```python
from build123d import *

# Parameters (mm, degrees)
SKETCH002_R     = 2.5
PAD002_DEPTH    = 7.5
SKETCH003_R     = 2.5
PAD003_DEPTH    = 7.25
SKETCH004_W     = 7.7928
SKETCH004_H     = 28.3985
PAD004_DEPTH    = 7
SKETCH006_W     = 20.21794
SKETCH006_H     = 4
POCKET_DEPTH    = 3
SKETCH_R        = 1.6
PAD_DEPTH       = 2
SKETCH001_W     = 53.9946
SKETCH001_H     = 28.4007
SKETCH001_W_2   = 44.2
SKETCH001_H_2   = 24.4007
PAD001_DEPTH    = 4
FILLET001_R     = 1
FILLET002_R     = 1
SKETCH007_W     = 4
SKETCH007_H     = 31.150972
POCKET001_DEPTH = 2


with BuildPart() as pad002:
    # Sketch002 → Pad002 (new body, symmetric)
    with BuildSketch(Plane(origin=(0.5, -2, 16), x_dir=(1, 0, 0), z_dir=(0, -0.707107, 0.707107))):
        with Locations((90.268963, -10.326332)):
            Circle(SKETCH002_R)
    extrude(amount=PAD002_DEPTH, both=True)


with BuildPart() as pad003:
    # Sketch003 → Pad003 (new body, symmetric)
    with BuildSketch(Plane(origin=(0, 8, 9), x_dir=(1, 0, 0), z_dir=(0, 0.707107, 0.707107))):
        with Locations((90.80912, 0.294413)):
            Circle(SKETCH003_R)
    extrude(amount=PAD003_DEPTH, both=True)


with BuildPart() as pocket:
    # Sketch004 → Pad004 (new body)
    with BuildSketch(Plane.XY.offset(6)):
        with Locations((90.6495, -0.51115)):
            Rectangle(SKETCH004_W, SKETCH004_H)
    extrude(amount=PAD004_DEPTH)

    # Cut: cut Pad003
    add(pad003.part, mode=Mode.SUBTRACT)

    # Cut001: cut Pad002
    add(pad002.part, mode=Mode.SUBTRACT)

    # Sketch006 → Pocket (cut)
    with BuildSketch(Plane(origin=(86.7531, 0, 0), x_dir=(0, -1, 0), z_dir=(-1, 0, 0))):
        with Locations((0.648237, 8.121586)):
            Rectangle(SKETCH006_W, SKETCH006_H)
    extrude(amount=-POCKET_DEPTH, mode=Mode.SUBTRACT)


with BuildPart() as pocket001:
    # Sketch → Pad (new body)
    with BuildSketch(Plane.XY):
        Polygon((21.7667, -25.4923), (21.7667, -16.53082), (30.29072, -16.53082), (30.29072, -21.52783), (40.54589, -21.52783), (40.54589, 20.48012), (30.54589, 20.48012), (30.54589, 15.49558), (21.7928, 15.49558), (21.7928, 24.4708), (44.46409, 24.4708), (44.46409, 13.68925), (70.02404, 13.68925), (70.02404, 24.4708), (76.4105, 24.4708), (76.4105, 13.68925), (94.54589, 13.68925), (94.54589, -14.71075), (76.26045, -14.71075), (76.26045, -25.4923), (69.87399, -25.4923), (69.87399, -14.71075), (44.43799, -14.71075), (44.43799, -25.4923), align=None)
        with Locations((25.98991, 19.9708)):
            Circle(SKETCH_R, mode=Mode.SUBTRACT)
        with Locations((25.99838, -21.01867)):
            Circle(SKETCH_R, mode=Mode.SUBTRACT)
        with Locations((72.97054, 20.01877)):
            Circle(SKETCH_R, mode=Mode.SUBTRACT)
        with Locations((72.94754, -21.05239)):
            Circle(SKETCH_R, mode=Mode.SUBTRACT)
    extrude(amount=PAD_DEPTH)

    # Sketch001 → Pad001 (new body)
    with BuildSketch(Plane.XY.offset(2)):
        with Locations((67.5478, -0.51015)):
            Rectangle(SKETCH001_W, SKETCH001_H)
        with Locations((64.6505, -0.51015)):
            Rectangle(SKETCH001_W_2, SKETCH001_H_2, mode=Mode.SUBTRACT)
    extrude(amount=PAD001_DEPTH)

    # Fusion: union Pocket
    add(pocket.part)

    # Fillet001
    fillet001_edges = [pocket001.edges().sort_by_distance(p)[0] for p in [
        (87.573856, -14.7104, 13),
        (93.844607, -14.7104, 13),
        (93.843844, 13.6881, 13),
        (87.614776, 13.6881, 13),
    ]]
    fillet(fillet001_edges, radius=FILLET001_R)

    # Fillet002
    fillet002_edges = [pocket001.edges().sort_by_distance(p)[0] for p in [
        (76.26045, -25.4923, 1),
        (69.87399, -25.4923, 1),
        (44.43799, -25.4923, 1),
        (21.7667, -25.4923, 1),
        (21.7928, 15.49558, 1),
        (21.7667, -16.53082, 1),
        (21.7928, 24.4708, 1),
        (70.02404, 24.4708, 1),
        (76.4105, 24.4708, 1),
        (44.46409, 24.4708, 1),
    ]]
    fillet(fillet002_edges, radius=FILLET002_R)

    # Sketch007 → Pocket001 (cut)
    with BuildSketch(Plane(origin=(0, 0, 0), x_dir=(1, 0, 0), z_dir=(0, 0, -1))):
        with Locations((50.046217, 0.273968)):
            Rectangle(SKETCH007_W, SKETCH007_H)
    extrude(amount=-POCKET001_DEPTH, mode=Mode.SUBTRACT)


solid = pocket001.part
```
Build history of the part. All positions in model axes, mm. A direction names the side the tool comes from. Coordinates: 2 decimals unless noted, no trailing zeros. Write each loop counter-clockwise with the first axis right and the second up, starting at its lowest first coordinate (ties: lowest second). Pieces come first, ordered by that corner, then holes.
1. Pull direction Y, two halves, no side cores. Call faces 1 (the flat face through (73, -25.492, 1)), 2 (the flat face through (91, 5, 6)), 3 (the flat face through (73, 18, 2)): released by +Y, released by -Y, zero draft, split by the parting line, or undercut.
Answer block:
face 1: released by -Y
face 2: undercut
face 3: zero draft
2. Drop flat-ended pins along their axis: pin 1 (1.6 mm diameter, centred on y = 18, z = 1.5, fed in from +X); pin 2 (1.8 mm diameter, centred on x = 90, z = 10, fed in from -Y); pin 3 (5 mm diameter, centred on x = 29.5, z = 6.5, fed in from -Y); pin 4 (6 mm diameter, centred on x = 68.5, y = 3.5, fed in from +Z). Give the stop position or say it passes through.
Answer block:
pin 1: stops at x = 76.41
pin 2: stops at y = -14.71
pin 3: passes through
pin 4: stops at z = 2
3. 3-axis set-ups, long thin cutter, end or side, ignore diameter. For faces 4 (the flat face through (42.55, -1, 4)), 5 (the flat face through (89.753, 0, 9)), 6 (the flat face through (86.753, -1, 11)), 7 (the flat face through (30.546, 18, 1)), 8 (the flat face through (69.874, -20, 1)): which of +Z, -Z, +X, -X, +Y, -Y reach the whole face in a straight line?
Answer block:
face 4: +Z
face 5: -X
face 6: +Z, -X, +Y, -Y
face 7: +Z, -Z
face 8: +Z, -Z, -Y
4. Band-saw the part on D-D, the plane z = 1. Give the number of separate pieces and of enclosed holes in the cut face, and give its area (3 significant figures).
Answer block:
separate pieces: 2
enclosed holes: 4
area: 1,840 mm2
5. Drill centre lines: probe 1 along X at (y, z) = (1.5, 1.75); probe 2 along Y at (x, z) = (74.5, 5.5); probe 3 along Y at (x, z) = (87, 7). Where is each one in solid material? Low to high.
Answer block:
probe 1: x = 40.55 to 48.05, 52.05 to 94.55
probe 2: y = -14.71 to -12.71, 11.69 to 13.69
probe 3: y = -14.71 to -10.76, 9.46 to 13.69
6. Band-saw the part on B-B, the plane x = 49. Give the cut face in (y, z).
Answer block:
outline: (-14.71, 2) - (-12.71, 2) - (-12.71, 6) - (-14.71, 6) - close; (11.69, 2) - (13.69, 2) - (13.69, 6) - (11.69, 6) - close
7. Band-saw the part on C-C, the plane x = 32. Give the cut face in (y, z), and give its area (3 significant figures).
Answer block:
outline: (-25.49, 0) - (-21.53, 0) - (-21.53, 2) - (-25.49, 2) - close; (20.48, 0) - (24.47, 0) - (24.47, 2) - (20.48, 2) - close
area: 15.9 mm2
